Here's how the part is built. I have some questions about the finished solid (model axes, mm). Coordinates: 2 decimals unless noted, no trailing zeros. Order: outer loops, then holes, each group sorted by start corner. A loop starts at its lowest first (then second) coordinate and runs counter-clockwise, first axis right, second up. Notation, with made-up numbers: (-33, 70.25) - (25, 70.25) arc R14 ccw to (25, 92.25) - close; hole circle Ø2 at (4, 65). An arc over 180 degrees is marked (long way). Answer as CSV lines item,"result". Start each with the question number.
Q1. For pin 1 Ø4 at (x, z) = (-203.2, 139.7) entering from -Y, with a flat end and sliding along its axis, tell me the tip position at first contact or that it passes through.
Q2. Suppose I cut it at B-B (y = -1.5). Count the separate pieces of the cut face and the enclosed holes in it, then the cut area to 3 significant figures.
Q3. Suppose I cut it at D-D (z = -101.6). Please give me the cut outline in (x, y), then the cut area to 3 significant figures.
Q4. Suppose I cut it at A-A (z = 101.6). Please give me the cut outline in (x, y).
Q5. Suppose I cut it at C-C (x = 165.1). Please give me the cut outline in (y, z), then the cut area to 3 significant figures.
Q6. Thinking about a two-plate mould opening in Z: for faces 1 (the face through (-3, 0, 2)), 2 (the face through (68.188, -2.348, -110.614)), which applies, released by +Z, released by -Z, zero draft, split by the parting line, or undercut?
Q7. I need wall thicknesses on line 1 (X direction, y = -1.8, z = 102.5); line 2 (X direction, y = -3.95, z = -136.5); line 3 (Z direction, x = -165.1, y = -3.05). Which ranges of each line are inside material? Lowest first, please.
from build123d import *

# Parameters (mm, degrees)
F0_W     = 431.8
F0_H     = 304.8
F0_R     = 3.4925
F0_R_2   = 10.16
F0_R_3   = 7.366
F1_DEPTH = 4.7625


with BuildPart() as f1:
    # F0 (on Front) → F1 (new body)
    with BuildSketch(Plane.XZ):
        Rectangle(F0_W, F0_H)
        with Locations((-203.2, -139.7)):
            Circle(F0_R, mode=Mode.SUBTRACT)
        with Locations((-165.1, -101.6)):
            Circle(F0_R_2, mode=Mode.SUBTRACT)
        with Locations((-63.5, -101.6)):
            Circle(F0_R_2, mode=Mode.SUBTRACT)
        with Locations((63.5, -101.6)):
            Circle(F0_R_2, mode=Mode.SUBTRACT)
        with Locations((203.2, -139.7)):
            Circle(F0_R, mode=Mode.SUBTRACT)
        with Locations((165.1, -101.6)):
            Circle(F0_R_2, mode=Mode.SUBTRACT)
        with Locations((-203.2, 0)):
            Circle(F0_R, mode=Mode.SUBTRACT)
        with Locations((-165.1, 0)):
            Circle(F0_R_3, mode=Mode.SUBTRACT)
        with Locations((-63.5, 0)):
            Circle(F0_R_3, mode=Mode.SUBTRACT)
        with Locations((-165.1, 101.6)):
            Circle(F0_R_3, mode=Mode.SUBTRACT)
        with Locations((-203.2, 139.7)):
            Circle(F0_R, mode=Mode.SUBTRACT)
        with Locations((-69.9898, 101.6)):
            Circle(F0_R_3, mode=Mode.SUBTRACT)
        with Locations((63.5, 0)):
            Circle(F0_R_2, mode=Mode.SUBTRACT)
        with Locations((165.1, 0)):
            Circle(F0_R_2, mode=Mode.SUBTRACT)
        with Locations((203.2, 0)):
            Circle(F0_R, mode=Mode.SUBTRACT)
        with Locations((63.5, 101.6)):
            Circle(F0_R_3, mode=Mode.SUBTRACT)
        with Locations((165.1, 101.6)):
            Circle(F0_R_3, mode=Mode.SUBTRACT)
        with Locations((203.2, 139.7)):
            Circle(F0_R, mode=Mode.SUBTRACT)
    extrude(amount=F1_DEPTH)


solid = f1.part
Here are the results:
1,pin 1,"passes through"
2,separate pieces,"1"
2,enclosed holes,"18"
2,area,"128,000 mm²"
3,outline,"(-215.9, -4.76) - (-175.26, -4.76) - (-175.26, 0) - (-215.9, 0) - close; (-154.94, -4.76) - (-73.66, -4.76) - (-73.66, 0) - (-154.94, 0) - close; (-53.34, -4.76) - (53.34, -4.76) - (53.34, 0) - (-53.34, 0) - close; (73.66, -4.76) - (154.94, -4.76) - (154.94, 0) - (73.66, 0) - close; (175.26, -4.76) - (215.9, -4.76) - (215.9, 0) - (175.26, 0) - close"
3,area,"1,670 mm²"
4,outline,"(-215.9, -4.76) - (-172.47, -4.76) - (-172.47, 0) - (-215.9, 0) - close; (-157.73, -4.76) - (-77.36, -4.76) - (-77.36, 0) - (-157.73, 0) - close; (-62.62, -4.76) - (56.13, -4.76) - (56.13, 0) - (-62.62, 0) - close; (70.87, -4.76) - (157.73, -4.76) - (157.73, 0) - (70.87, 0) - close; (172.47, -4.76) - (215.9, -4.76) - (215.9, 0) - (172.47, 0) - close"
5,outline,"(-4.76, -152.4) - (0, -152.4) - (0, -111.76) - (-4.76, -111.76) - close; (-4.76, -91.44) - (0, -91.44) - (0, -10.16) - (-4.76, -10.16) - close; (-4.76, 10.16) - (0, 10.16) - (0, 94.23) - (-4.76, 94.23) - close; (-4.76, 108.97) - (0, 108.97) - (0, 152.4) - (-4.76, 152.4) - close"
5,area,"1,190 mm²"
6,face 1,"zero draft"
6,face 2,"undercut"
7,line 1,"x = -215.9 to -172.41, -157.79 to -77.3, -62.68 to 56.19, 70.81 to 157.79, 172.41 to 215.9"
7,line 2,"x = -215.9 to -204.6, -201.8 to 201.8, 204.6 to 215.9"
7,line 3,"z = -152.4 to -111.76, -91.44 to -7.37, 7.37 to 94.23, 108.97 to 152.4"
